from build123d import *

# Parameters (mm, degrees)
F0_W     = 3
F0_H     = 6
F0_R     = 6.75
F1_DEPTH = 3


with BuildPart() as f1:
    # F0 (on Front) → F1 (new body)
    with BuildSketch(Plane.XZ):
        with BuildLine():
            Line((-62.884246, -24.944276), (-33.535898, -8))
            Line((-33.535898, -8), (27, -8))
            ThreePointArc((27, -8), (29.837722, -9.486833), (33, -10))
            ThreePointArc((33, -10), (36.868919, -9.221251), (40.135255, -7.006293))
            Line((40.135255, -7.006293), (61.78589, -19.506293))
            Line((61.78589, -19.506293), (64.28589, -15.176166))
            Line((64.28589, -15.176166), (42.635255, -2.676166))
            ThreePointArc((42.635255, -2.676166), (40.961208, 6.051378), (33, 10))
            ThreePointArc((33, 10), (29.837722, 9.486833), (27, 8))
            Line((27, 8), (-33, 8))
            ThreePointArc((-33, 8), (-37.658743, 7.386665), (-42, 5.588457))
            Line((-42, 5.588457), (-70.578838, -10.911543))
            ThreePointArc((-70.578838, -10.911543), (-73.149015, -12.7112), (-75.367638, -14.929823))
            Line((-75.367638, -14.929823), (-90.722898, -33.229509))
            ThreePointArc((-90.722898, -33.229509), (-78.192339, -36.056949), (-66.967653, -29.810691))
            Line((-66.967653, -29.810691), (-62.884246, -24.944276))
        make_face()
        with Locations((-33, 0)):
            Rectangle(F0_W, F0_H, mode=Mode.SUBTRACT)
        with Locations((33, 0)):
            Circle(F0_R, mode=Mode.SUBTRACT)
    extrude(amount=F1_DEPTH)


solid = f1.part
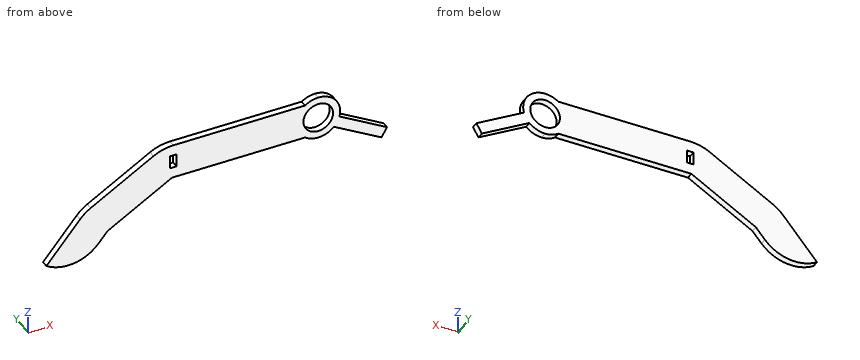
Verification items for the finished model (mm, model axes). Give positions to 0.01 mm unless a question says otherwise; leave off trailing zeros. Write each loop counter-clockwise with the first axis right and the second up, starting at its lowest first coordinate (ties: lowest second). Pieces come first, ordered by that corner, then holes. Notation, with made-up numbers: M 24,-16 L 67,-16 A30 cw 67,13 Z; hole C 58,50.25 d7. An arc over 180 degrees is marked long. Write item = value, one per line.
(1) Sectioned sample at B-B (z = 0). Record the cut outline in (x, y), then the cut area to 3 significant figures.
Found:
outline = M -51.68,-3 L -34.5,-3 L -34.5,0 L -51.68,0 Z; M -31.5,-3 L 26.25,-3 L 26.25,0 L -31.5,0 Z; M 39.75,-3 L 43,-3 L 43,0 L 39.75,0 Z
area = 235 mm2
(2) Material ranges on line 1 (Z direction, x = 33, y = -1.55); line 2 (X direction, y = -2.1, z = -2.5); line 3 (X direction, y = -2.5, z = -2), recorded low to high.
Found:
line_1 = -10 to -6.75, 6.75 to 10
line_2 = -56.01 to -34.5, -31.5 to 26.73, 39.27 to 42.68
line_3 = -55.14 to -34.5, -31.5 to 26.55, 39.45 to 42.8
(3) Sectioned sample at C-C (x = -23.5). Record the cut outline in (y, z).
Found:
outline = M -3,-8 L 0,-8 L 0,8 L -3,8 Z
(4) Go/stop test with flat-tipped pins: pin 1 Ø1.5 at (x, y) = (36, -1) entering from +Z; pin 2 Ø1.5 at (y, z) = (-1, -0.5) entering from -X; pin 3 Ø0.9 at (y, z) = (-2, 1.5) entering from +X. Record where each tip stops, or that it passes through.
Found:
pin_1 = 9.74
pin_2 = -53.84
pin_3 = 42.94
(5) Sectioned sample at D-D (z = -23). Record the cut outline in (x, y), then the cut area to 3 significant figures.
Found:
outline = M -82.14,-3 L -59.52,-3 L -59.52,0 L -82.14,0 Z
area = 67.9 mm2
(6) Sectioned sample at A-A (y = -1.9). Record the cut outline in (x, z).
Found:
outline = M -90.72,-33.23 A18 ccw -66.97,-29.81 L -62.88,-24.94 L -33.54,-8 L 27,-8 A10 ccw 33,-10 A10 ccw 40.14,-7.01 L 61.79,-19.51 L 64.29,-15.18 L 42.64,-2.68 A10 ccw 33,10 A10 ccw 27,8 L -33,8 A18 ccw -42,5.59 L -70.58,-10.91 A18 ccw -75.37,-14.93 Z; hole M -34.5,-3 L -31.5,-3 L -31.5,3 L -34.5,3 Z; hole C 33,0 d13.5
